from build123d import *

# Parameters (mm, degrees)
SKETCH_W   = 407
SKETCH_H   = 495
SKETCH_R   = 1.8
SKETCH_R_2 = 2.4
PAD_DEPTH  = 8


with BuildPart() as part:
    # Sketch → Pad (new body)
    with BuildSketch(Plane.XY):
        Rectangle(SKETCH_W, SKETCH_H)
        with Locations((-190.5, 234.5)):
            Circle(SKETCH_R, mode=Mode.SUBTRACT)
        with Locations((190.5, 234.5)):
            Circle(SKETCH_R, mode=Mode.SUBTRACT)
        with Locations((-190.5, -234.5)):
            Circle(SKETCH_R, mode=Mode.SUBTRACT)
        with Locations((190.5, -234.5)):
            Circle(SKETCH_R, mode=Mode.SUBTRACT)
        with Locations((190.5, 55.9)):
            Circle(SKETCH_R_2, mode=Mode.SUBTRACT)
        with BuildLine():
            ThreePointArc((-143.5, -147.5), (-178.5, -182.5), (-143.5, -217.5))
            Line((-143.5, -217.5), (-43.5, -217.5))
            ThreePointArc((-43.5, -217.5), (-8.5, -182.5), (-43.5, -147.5))
            Line((-143.5, -147.5), (-43.5, -147.5))
        make_face(mode=Mode.SUBTRACT)
    extrude(amount=PAD_DEPTH)


solid = part.part
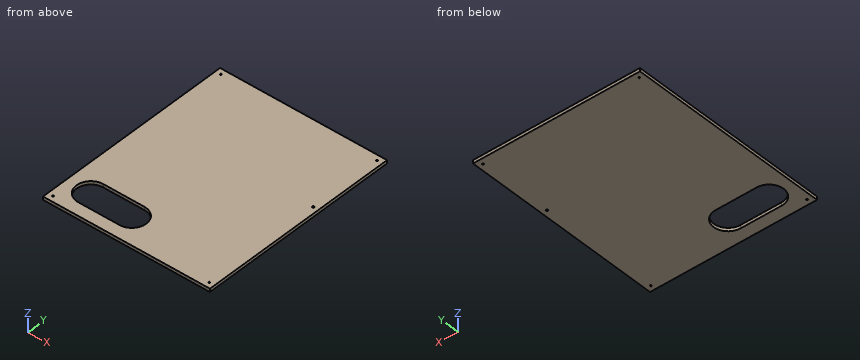
Design review of the part built by this model. Coordinates are the model's own, in mm. Round coordinates to 2 decimals unless told otherwise and drop trailing zeros. Write each loop counter-clockwise with the first axis right and the second up, starting at its lowest first coordinate (ties: lowest second). Pieces come first, ordered by that corner, then holes. Notation, with made-up numbers: (62.25, -19.75) -> (115.25, -19.75) arc R18 cw to (115.25, 14.25) -> close; hole circle Ø11 at (-37, -3.75). An arc over 180 degrees is marked (long way). One line per item, written item: value. Start each with the question number.
Q1. Add section A-A (x = -90). Give the boundary of the cut face in (y, z), then the cut area to 3 significant figures.
Q2. To check wall thickness, follow probe 1 along Y at (x, z) = (190.5, 4.25); probe 2 along Y at (x, z) = (-190.5, 3.5); probe 3 along X at (y, z) = (234.5, 4). State the ranges of each line that lie inside material, in increasing order.
Q3. Add section C-C (z = 2.5). Give the boundary of the cut face in (x, y).
Q4. Add section B-B (y = -182.5). Give the boundary of the cut face in (x, z).
Q5. Insertion check: P1, Ø2, axis at x = 190.5, y = 234.5, coming from the -Z side. The pin has a flat end and moves straight along its axis. Give the tip position at first contact, or say it passes through.
Response:
1. outline: (-247.5, 0) -> (-217.5, 0) -> (-217.5, 8) -> (-247.5, 8) -> close; (-147.5, 0) -> (247.5, 0) -> (247.5, 8) -> (-147.5, 8) -> close
1. area: 3,400 mm^2
2. probe 1: y = -247.5 to -236.3, -232.7 to 53.5, 58.3 to 232.7, 236.3 to 247.5
2. probe 2: y = -247.5 to -236.3, -232.7 to 232.7, 236.3 to 247.5
2. probe 3: x = -203.5 to -192.3, -188.7 to 188.7, 192.3 to 203.5
3. outline: (-203.5, -247.5) -> (203.5, -247.5) -> (203.5, 247.5) -> (-203.5, 247.5) -> close; hole circle Ø3.6 at (-190.5, -234.5); hole circle Ø3.6 at (-190.5, 234.5); hole (-143.5, -217.5) -> (-43.5, -217.5) arc R35 ccw to (-43.5, -147.5) -> (-143.5, -147.5) arc R35 ccw to start; hole circle Ø4.8 at (190.5, 55.9); hole circle Ø3.6 at (190.5, -234.5); hole circle Ø3.6 at (190.5, 234.5)
4. outline: (-203.5, 0) -> (-178.5, 0) -> (-178.5, 8) -> (-203.5, 8) -> close; (-8.5, 0) -> (203.5, 0) -> (203.5, 8) -> (-8.5, 8) -> close
5. P1: passes through
